from build123d import *

# Parameters (mm, degrees)
CROQUIS1_W              = 12.7
CROQUIS1_H              = 25
CROQUIS1_H_2            = 5
CROQUIS1_W_2            = 15
CROQUIS1_H_3            = 15
SALIENTE_EXTRUIR1_DEPTH = 20
CROQUIS2_R              = 4
CORTAR_EXTRUIR1_DEPTH   = 12.7


with BuildPart() as part:
    # Croquis1 → Saliente-Extruir1 (new body)
    # profile 1 of 6: a face of its own
    with BuildSketch(Plane(origin=(0, 0, 0), x_dir=(1, 0, 0), z_dir=(0, 1, 0))):
        Polygon((-117.3, -20), (130, -20), (130, 20), (-117.3, 20), (-117.3, 15), (-130, 15), (-130, 7.5), (-130, -7.5), (-130, -15), (-117.3, -15), align=None)
        with BuildLine():
            ThreePointArc((110, 7.5), (117.5, 0), (110, -7.5))
            Line((110, -7.5), (-110, -7.5))
            ThreePointArc((-110, -7.5), (-117.5, 0), (-110, 7.5))
            Line((-110, 7.5), (110, 7.5))
        make_face(mode=Mode.SUBTRACT)
    # profile 2 of 6: a face of its own
    with BuildSketch(Plane(origin=(0, 0, 0), x_dir=(1, 0, 0), z_dir=(0, 1, 0))):
        with Locations((-123.65, -32.5)):
            Rectangle(CROQUIS1_W, CROQUIS1_H)
    # profile 3 of 6: a face of its own
    with BuildSketch(Plane(origin=(0, 0, 0), x_dir=(1, 0, 0), z_dir=(0, 1, 0))):
        with Locations((-123.65, -17.5)):
            Rectangle(CROQUIS1_W, CROQUIS1_H_2)
    # profile 4 of 6: a face of its own
    with BuildSketch(Plane(origin=(0, 0, 0), x_dir=(1, 0, 0), z_dir=(0, 1, 0))):
        with Locations((-123.65, 17.5)):
            Rectangle(CROQUIS1_W, CROQUIS1_H_2)
    # profile 5 of 6: a face of its own
    with BuildSketch(Plane(origin=(0, 0, 0), x_dir=(1, 0, 0), z_dir=(0, 1, 0))):
        with Locations((-123.65, 32.5)):
            Rectangle(CROQUIS1_W, CROQUIS1_H)
    # profile 6 of 6: a face of its own
    with BuildSketch(Plane(origin=(0, 0, 0), x_dir=(1, 0, 0), z_dir=(0, 1, 0))):
        with Locations((-137.5, 0)):
            Rectangle(CROQUIS1_W_2, CROQUIS1_H_3)
    extrude(amount=SALIENTE_EXTRUIR1_DEPTH)

    # Croquis2 → Cortar-Extruir1 (cut)
    with BuildSketch(Plane.ZY.offset(130)):
        with Locations((-35, 10)):
            Circle(CROQUIS2_R)
        with Locations((35, 10)):
            Circle(CROQUIS2_R)
    extrude(amount=-CORTAR_EXTRUIR1_DEPTH, mode=Mode.SUBTRACT)


solid = part.part
Can you work these out from the model? Positions are in its coordinate system, mm. A direction names the side the tool comes from. Give positions to 0.01 mm unless a question says otherwise; leave off trailing zeros. Loops run counter-clockwise (first coordinate to the right, second up) from the corner with the lowest first, then second, coordinate; pieces in that order, holes last. Notation, with made-up numbers: M 42,57.5 L 79,57.5 A28 ccw 79,81.5 Z; hole C -21.75,17.5 d8. An arc over 180 degrees is marked long. One line per item, written item: value. Start each with the question number.
1) If we section it at A-A, the plane z = -35: Write out the boundary of the cut face in (x, y).
2) If I drill on line 1 (Z direction, x = 69, y = 10); line 2 (Y direction, x = -125, z = -35); line 3 (X direction, y = 2.25, z = -38.5), over which ranges is the centre line in solid material (lowest first)? Write a range as [from, to].
3) If we section it at D-D, the plane z = 17: Write out the boundary of the cut face in (x, y), and give its area (3 significant figures).
4) If we section it at C-C, the plane x = 14: Write out the boundary of the cut face in (y, z).
5) If we section it at B-B, the plane y = 10: Write out the boundary of the cut face in (x, z).
6) On a 3-axis mill with a long thin cutter (end or side, diameter ignored), from which of +Z, -Z, +X, -X, +Y, -Y can I reach the whole of each face in a straight line? I mean faces 4 (the face through (-130, 10, -27)), 5 (the face through (117.5, 9.86, -0.16)), 6 (the face through (-117.3, 10, -30)), 7 (the face through (-138, 10, 7.5)). Say none if no direction works.
7) Thinking about a two-plate mould opening in Y: for faces 1 (the face through (5, 10, 20)), 2 (the face through (-124, 10, 31)), 3 (the face through (-8, 20, 13)), which applies, +Y half, -Y half, draft (parallel to the pull), parting line (faces both ways), or undercut?
8) I'm going to push flat-ended pins straight in: pin 1 (6 mm diameter, centred on x = 63, y = 14, fed in from +Z); pin 2 (10 mm diameter, centred on y = 9, z = 36.5, fed in from +X); pin 3 (4.5 mm diameter, centred on x = -136, y = 11.5, fed in from -Z); pin 4 (10 mm diameter, centred on x = 10.5, z = 1.5, fed in from +Y). Where does each tip first touch, or does it pass through?
Completed:
1. outline: M -130,0 L -117.3,0 L -117.3,6 L -130,6 Z; M -130,14 L -117.3,14 L -117.3,20 L -130,20 Z
2. line 1: z = [-20, -7.5], [7.5, 20]
2. line 2: y = [0, 6], [14, 20]
2. line 3: x = [-130, -117.3]
3. outline: M -130,0 L 130,0 L 130,20 L -130,20 Z
3. area: 5,200 mm^2
4. outline: M 0,-20 L 20,-20 L 20,-7.5 L 0,-7.5 Z; M 0,7.5 L 20,7.5 L 20,20 L 0,20 Z
5. outline: M -145,-7.5 L -130,-7.5 L -130,-31 L -117.3,-31 L -117.3,-20 L 130,-20 L 130,20 L -117.3,20 L -117.3,31 L -130,31 L -130,7.5 L -145,7.5 Z; M -130,-45 L -117.3,-45 L -117.3,-39 L -130,-39 Z; M -130,39 L -117.3,39 L -117.3,45 L -130,45 Z; hole M -110,-7.5 L 110,-7.5 A7.5 ccw 110,7.5 L -110,7.5 A7.5 ccw Z
6. face 4: -Z, -X, +Y, -Y
6. face 5: +Y, -Y
6. face 6: -Z, +X, +Y, -Y
6. face 7: +Z, -X, +Y, -Y
7. face 1: draft
7. face 2: undercut
7. face 3: +Y half
8. pin 1: stops at z = 20
8. pin 2: stops at x = -117.3
8. pin 3: stops at z = -7.5
8. pin 4: passes through
